Read the model definition and answer for the solid it produces. Units are mm, in the model's axes. Face numbers are marked on the shaded views. A direction names the side the tool comes from. Coordinates: 2 decimals unless noted, no trailing zeros. Loops run counter-clockwise (first coordinate to the right, second up) from the corner with the lowest first, then second, coordinate; pieces in that order, holes last.
Q1. Which of the six approach directions +Z, -Z, +X, -X, +Y, -Y give full straight-line access (tool end or side, diameter ignored) to the marked faces 5, 6, 7 and 8?
Q2. The mould has two halves that part along X. Classify the marked faces 1, 2, 3 and 4: pulls with the +X half, pulls with the -X half, needs draft (parallel to the pull), parting line crosses it, or undercut.
Q3. Section D-D (z = -6.25) is taken. Give the vertices of the cut face in (x, y).
Q4. Section A-A (z = -12) is taken. Give the vertices of the cut face in (x, y).
Q5. Section B-B (y = 7) is taken. Give the vertices of the cut face in (x, z), then the cut area to 3 significant figures.
Q6. Flat-ended cylindrical pins translate along their axes: P1, Ø10, axis at x = 2, y = -2, coming from the -Z side; P2, Ø5, axis at x = 2.5, y = 9, coming from the -Z side; P3, Ø10, axis at y = 6.5, z = -7, coming from the +X side. Find the tip coordinate at first contact, or state that the pin passes through.
Q7. Straight lines are drawn through the part: line 1 (Z direction, x = -4.75, y = -4.5); line 2 (Y direction, x = 3, z = 5); line 3 (Y direction, x = -3, z = 6.75). For each, find the intervals that lie inside material, in ascending order.
Q8. Section C-C (z = -1) is taken. Give the vertices of the cut face in (x, y).
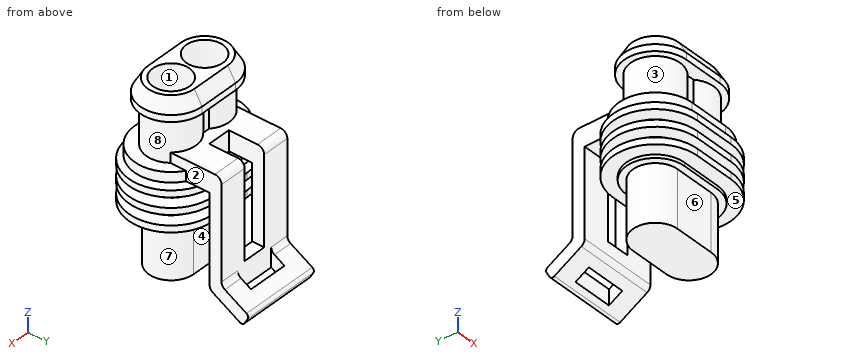
from build123d import *
from OCP.BRepFilletAPI import BRepFilletAPI_MakeChamfer

# Parameters (mm, degrees)
SKETCH1_R          = 2.75
EXTRUDE1_DEPTH     = 6.5
SKETCH2_R          = 2.75
EXTRUDE2_DEPTH     = 3
CHAMFER1_SIZE      = 2
CHAMFER1_SIZE2     = 1.154700538
SKETCH4_R          = 2.75
EXTRUDE3_DEPTH     = 1.5
EXTRUDE4_DEPTH     = 5.9
EXTRUDE5_DEPTH     = 15.5
CUT_EXTRUDE1_DEPTH = 3
CUT_EXTRUDE2_DEPTH = 1.75


with BuildPart() as part:
    # Sketch1 → Extrude1 (new body)
    with BuildSketch(Plane.XY):
        with BuildLine():
            Line((0.524621241, 2.75), (-0.524621241, 2.75))
            ThreePointArc((-0.524621241, 2.75), (-6.7, 0), (-0.524621241, -2.75))
            Line((-0.524621241, -2.75), (0.524621241, -2.75))
            ThreePointArc((0.524621241, -2.75), (6.7, 0), (0.524621241, 2.75))
        make_face()
        with Locations(Location((3, 0, 0), (0, 0, 180))):
            Circle(SKETCH1_R, mode=Mode.SUBTRACT)
        with Locations(Location((-3, 0, 0), (0, 0, 180))):
            Circle(SKETCH1_R, mode=Mode.SUBTRACT)
    extrude(amount=EXTRUDE1_DEPTH)

    # Sketch2 → Extrude2 (add)
    with BuildSketch(Plane.XY.offset(6.5)):
        with BuildLine():
            Line((3, 4.65), (-3, 4.65))
            ThreePointArc((-3, 4.65), (-7.65, 0), (-3, -4.65))
            Line((-3, -4.65), (3, -4.65))
            ThreePointArc((3, -4.65), (7.65, 0), (3, 4.65))
        make_face()
        with Locations(Location((3, 0, 0), (0, 0, 180))):
            Circle(SKETCH2_R, mode=Mode.SUBTRACT)
        with Locations(Location((-3, 0, 0), (0, 0, 180))):
            Circle(SKETCH2_R, mode=Mode.SUBTRACT)
    extrude(amount=EXTRUDE2_DEPTH)

    # Chamfer1: one chamfer whose edges measure the first distance from different faces: ONE call of the kernel's chamfer builder (chamfer() names one face for all edges)
    chamfer1_edges_1 = [part.edges().sort_by_distance(p)[0] for p in [
        (7.65, 0, 9.5),
    ]]
    chamfer1_side_1 = [part.faces().sort_by_distance(p)[0] for p in [
        (7.65, 0, 8),
    ]]
    chamfer1_edges_2 = [part.edges().sort_by_distance(p)[0] for p in [
        (0, 4.65, 9.5),
    ]]
    chamfer1_side_2 = [part.faces().sort_by_distance(p)[0] for p in [
        (0, 4.65, 8),
    ]]
    chamfer1_edges_3 = [part.edges().sort_by_distance(p)[0] for p in [
        (-7.65, 0, 9.5),
    ]]
    chamfer1_side_3 = [part.faces().sort_by_distance(p)[0] for p in [
        (-7.65, 0, 8),
    ]]
    chamfer1_edges_4 = [part.edges().sort_by_distance(p)[0] for p in [
        (0, -4.65, 9.5),
    ]]
    chamfer1_side_4 = [part.faces().sort_by_distance(p)[0] for p in [
        (0, -4.65, 8),
    ]]
    chamfer1 = BRepFilletAPI_MakeChamfer(part.part.solid().wrapped)
    for e in chamfer1_edges_1:
        chamfer1.Add(CHAMFER1_SIZE, CHAMFER1_SIZE2, e.wrapped, chamfer1_side_1[0].wrapped)  # the first distance lies on this face
    for e in chamfer1_edges_2:
        chamfer1.Add(CHAMFER1_SIZE, CHAMFER1_SIZE2, e.wrapped, chamfer1_side_2[0].wrapped)  # the first distance lies on this face
    for e in chamfer1_edges_3:
        chamfer1.Add(CHAMFER1_SIZE, CHAMFER1_SIZE2, e.wrapped, chamfer1_side_3[0].wrapped)  # the first distance lies on this face
    for e in chamfer1_edges_4:
        chamfer1.Add(CHAMFER1_SIZE, CHAMFER1_SIZE2, e.wrapped, chamfer1_side_4[0].wrapped)  # the first distance lies on this face
    add(Compound.cast(chamfer1.Shape()), mode=Mode.REPLACE)

    # Sketch4 → Extrude3 (add)
    with BuildSketch(Plane(origin=(0, 0, 0), x_dir=(-1, 0, 0), z_dir=(0, 0, -1))):
        with BuildLine():
            Line((3, 5.5), (-3, 5.5))
            ThreePointArc((-3, 5.5), (-8.5, 0), (-3, -5.5))
            Line((-3, -5.5), (3, -5.5))
            ThreePointArc((3, -5.5), (8.5, 0), (3, 5.5))
        make_face()
        with Locations((3, 0)):
            Circle(SKETCH4_R, mode=Mode.SUBTRACT)
        with Locations((-3, 0)):
            Circle(SKETCH4_R, mode=Mode.SUBTRACT)
    extrude(amount=EXTRUDE3_DEPTH)

    # Sketch5 → Extrude4 (add, symmetric)
    with BuildSketch(Plane(origin=(0, 0, 0), x_dir=(0, 0, -1), z_dir=(1, 0, 0))):
        with BuildLine():
            Line((1.5, 0), (1.5, 8.2))
            Line((1.5, 8.2), (14.628718708, 8.2))
            ThreePointArc((14.628718708, 8.2), (15.128718708, 8.333974596), (15.494744112, 8.7))
            Line((15.494744112, 8.7), (17.833012702, 12.75))
            ThreePointArc((17.833012702, 12.75), (17.882962913, 13.129409523), (17.65, 13.433012702))
            Line((17.65, 13.433012702), (16.783974596, 13.933012702))
            ThreePointArc((16.783974596, 13.933012702), (16.404565074, 13.982962913), (16.100961894, 13.75))
            Line((16.100961894, 13.75), (14.224573519, 10.5))
            ThreePointArc((14.224573519, 10.5), (13.858548116, 10.133974596), (13.358548116, 10))
            Line((13.358548116, 10), (-0.5, 10))
            ThreePointArc((-0.5, 10), (-1.207106781, 9.707106781), (-1.5, 9))
            Line((-1.5, 9), (-1.5, 0))
            Line((-1.5, 0), (1.5, 0))
        make_face()
    extrude(amount=EXTRUDE4_DEPTH, both=True)

    # Sketch6 → Extrude5 (add)
    with BuildSketch(Plane(origin=(0, 0, -1.5), x_dir=(-1, 0, 0), z_dir=(0, 0, -1))):
        with BuildLine():
            Line((-3, 3.35), (3, 3.35))
            ThreePointArc((3, 3.35), (6.35, 0), (3, -3.35))
            Line((3, -3.35), (-3, -3.35))
            ThreePointArc((-3, -3.35), (-6.35, 0), (-3, 3.35))
        make_face()
    extrude(amount=EXTRUDE5_DEPTH)

    # Sketch10 → Cut-Extrude1 (cut, symmetric)
    with BuildSketch(Plane(origin=(0, 0, 0), x_dir=(0, 0, -1), z_dir=(1, 0, 0))):
        Polygon((17.4, 12), (15.090598923, 12), (13.358548116, 10), (16.245299462, 10), align=None)
    extrude(amount=CUT_EXTRUDE1_DEPTH, both=True, mode=Mode.SUBTRACT)

    # Sketch11 → Cut-Extrude2 (cut, symmetric)
    with BuildSketch(Plane(origin=(0, 0, 0), x_dir=(0, 0, -1), z_dir=(1, 0, 0))):
        Polygon((1.5, 4.673328578), (-1.5, 4.673328578), (-1.5, 10), (12.7, 10), (12.7, 8.2), (1.5, 8.2), align=None)
    extrude(amount=CUT_EXTRUDE2_DEPTH, both=True, mode=Mode.SUBTRACT)

    # Bælg: sweep along a path in Sketch8
    with BuildLine(Plane(origin=(0, 0, -1.5), x_dir=(-1, 0, 0), z_dir=(0, 0, -1))) as b_lg_path:
        Line((3, 3.35), (-3, 3.35))
        ThreePointArc((-3, 3.35), (-6.35, 0), (-3, -3.35))
        Line((-3, -3.35), (3, -3.35))
        ThreePointArc((3, -3.35), (6.35, 0), (3, 3.35))
    # Sketch7 → Bælg (sweep)
    with BuildSketch(Plane(origin=(0, 0, 0), x_dir=(0, 0, -1), z_dir=(1, 0, 0))):
        Polygon((8.5, 3.35), (1.5, 3.35), (1.5, 4.35), (2, 4.35), (2, 6.35), (3, 6.35), (3, 4.35), (4.5, 4.35), (4.5, 6.35), (5.5, 6.35), (5.5, 4.35), (7, 4.35), (7, 6.35), (8, 6.35), (8, 4.35), (8.5, 4.35), align=None)
    sweep(path=b_lg_path.line)


solid = part.part
Numbers:
1. face 5: -Z
1. face 6: -Z, +X, -X, -Y
1. face 7: -Z, +X
1. face 8: none
2. face 1: undercut
2. face 2: pulls with the +X half
2. face 3: undercut
2. face 4: needs draft
3. outline: (-5.9, 8.2) - (-1.75, 8.2) - (-1.75, 10) - (-5.9, 10) - close; (-3, -4.35) - (3, -4.35) arc R4.35 ccw to (3, 4.35) - (-3, 4.35) arc R4.35 ccw to start; (1.75, 8.2) - (5.9, 8.2) - (5.9, 10) - (1.75, 10) - close
4. outline: (-5.9, 8.2) - (-1.75, 8.2) - (-1.75, 10) - (-5.9, 10) - close; (-3, -3.35) - (3, -3.35) arc R3.35 ccw to (3, 3.35) - (-3, 3.35) arc R3.35 ccw to start; (1.75, 8.2) - (5.9, 8.2) - (5.9, 10) - (1.75, 10) - close
5. outline: (-5.9, -1.5) - (-1.75, -1.5) - (-1.75, 1.5) - (-5.9, 1.5) - close; (1.75, -1.5) - (5.9, -1.5) - (5.9, 1.5) - (1.75, 1.5) - close
5. area: 24.9 mm2
6. P1: stops at z = -17
6. P2: stops at z = -17.08
6. P3: stops at x = 9.17
7. line 1: z = -8 to -7, -5.5 to -4.5, -3 to -2, -1.5 to 0
7. line 2: y = -3.7 to -2.75, 2.75 to 3.7
7. line 3: y = -4.65 to -2.75, 2.75 to 4.65
8. outline: (-5.9, 4.67) arc R5.5 ccw to (-3, -5.5) - (3, -5.5) arc R5.5 ccw to (5.9, 4.67) - (5.9, 10) - (1.75, 10) - (1.75, 4.67) - (-1.75, 4.67) - (-1.75, 10) - (-5.9, 10) - close; hole (-5.75, 0) arc R2.75 ccw to (-0.25, 0) - close; hole (0.25, 0) arc R2.75 ccw to (5.75, 0) - close
